Here's how the part is built. I have some questions about the finished solid (model axes, mm). Round coordinates to 2 decimals unless told otherwise and drop trailing zeros. Write each loop counter-clockwise with the first axis right and the second up, starting at its lowest first coordinate (ties: lowest second). Pieces come first, ordered by that corner, then holes. Notation, with made-up numbers: M 37,77.25 L 72,77.25 A20 cw 72,99.25 Z; hole C 52,33 d8. An arc over 180 degrees is marked long. Use a Markdown table: item, result. Add a question column.
```python
from build123d import *

# Parameters (mm, degrees)
F3_D            = 3.81
F3_CSINK_D      = 4.318
F3_CSINK_ANGLE  = 90
F3_COPIES_COUNT = 8
F4_SIZE2        = 0.381
F4_SIZE         = 0.381


# Not quite as in the source:
# - a pattern or mirror of a feature is missing from the dataset's text; its kind, count and spacing are read off the source's solid


with BuildPart() as f1:
    # F0 (on Front) → F1 (revolve)
    with BuildSketch(Plane.XZ):
        with BuildLine():
            Line((12.7, 19.05), (11.4554, 19.05))
            Line((11.4554, 19.05), (11.4554, 0))
            Line((11.4554, 0), (22.225, 0))
            Line((22.225, 0), (22.225, 5.588))
            Line((22.225, 5.588), (15.875, 5.588))
            ThreePointArc((15.875, 5.588), (13.6299359697, 6.5179359697), (12.7, 8.763))
            Line((12.7, 8.763), (12.7, 19.05))
        make_face()
    revolve(axis=Axis((0, 0, -8.7907983398), (0, 0, -1)))

    # F3 (through all)
    with Locations(Plane.XY.offset(5.588)):
        with Locations((-19.05, 0)):
            f3 = CounterSinkHole(F3_D / 2, F3_CSINK_D / 2, counter_sink_angle=F3_CSINK_ANGLE)

    # F3_copies: F3 ×8 about axis
    f3_copies_axis = Axis((0, 0, 0), (0, 0, 1))
    for i in range(1, F3_COPIES_COUNT):
        add(f3.rotate(f3_copies_axis, i * 360 / F3_COPIES_COUNT), mode=Mode.SUBTRACT)

    # F4
    f4_edges = [f1.edges().sort_by_distance(p)[0] for p in [
        (-22.225, 0, 5.588),
        (-22.225, 0, 0),
        (-11.4554, 0, 0),
    ]]
    chamfer(f4_edges, length=F4_SIZE, length2=F4_SIZE2)


solid = f1.part
```
Item 1: If we mould it in two halves opening along Y, with no side actions, what happens to faces 1 (the face through (-2.75, 12.4, 13.98)), 2 (the face through (-9, 9, 0)), 3 (the face through (-15.16, -14.35, 2.63))? For each: +Y half, -Y half, draft (parallel to the pull), parting line (faces both ways), or undercut.
Item 2: For pin 1 Ø6 at (y, z) = (11, 9) entering from -X; pin 2 Ø6 at (x, y) = (-19.05, 0) entering from +Z; pin 3 Ø3.5 at (x, y) = (-13.47, -13.47) entering from +Z; pin 4 Ø3 at (x, z) = (-5.5, 10) entering from -Y, each with a flat end and sliding along its axis, tell me the tip position at first contact or that it passes through.
Item 3: Imagine slicing it at A-A on y = 0. Count the separate pieces of the cut face and the enclosed holes in it, plus the area to 3 significant figures.
Item 4: Imagine slicing it at D-D on z = 16. List the corners of the cut face in (x, y) for me.
Item 5: I need wall thicknesses on probe 1 along X at (y, z) = (0, 3.85) (3 decimals); probe 2 along Y at (x, z) = (0, 14.75); probe 3 along X at (y, z) = (19.05, 2.35) (3 decimals). Which ranges of each line are inside material? Lowest first, please. Write a range as from..to.
The answers:
| question | item | result |
|---|---|---|
| 1 | face 1 | parting line |
| 1 | face 2 | draft |
| 1 | face 3 | undercut |
| 2 | pin 1 | x = -9.95 |
| 2 | pin 2 | z = 5.59 |
| 2 | pin 3 | through |
| 2 | pin 4 | y = -12.05 |
| 3 | separate pieces | 4 |
| 3 | enclosed holes | 0 |
| 3 | area | 115 mm² |
| 4 | outline | C 0,0 d25.4; hole C 0,0 d22.91 |
| 5 | probe 1 | -22.225..-20.955, -17.145..-11.455, 11.455..17.145, 20.955..22.225 |
| 5 | probe 2 | -12.7..-11.46, 11.46..12.7 |
| 5 | probe 3 | -11.448..-1.905, 1.905..11.448 |
